from build123d import *

# Parameters (mm, degrees)
F0_W     = 4.7625
F0_H     = 3.175
F0_W_2   = 25.4
F0_H_2   = 4.7625
F1_DEPTH = 4.7625
F2_DEPTH = 25.4
F3_SIZE  = 6.35
F4_R     = 3.96875
F4_R_2   = 1.984375
F5_DEPTH = 0.79375
F6_DEPTH = 4.7625


with BuildPart() as f1:
    # F0 (on Top) → F1 (new body)
    with BuildSketch(Plane.XY):
        with Locations((27.78125, 17.0815)):
            Rectangle(F0_W, F0_H)
        with Locations((27.78125, -17.0815)):
            Rectangle(F0_W, F0_H)
        with Locations((-42.8625, -21.05025)):
            Rectangle(F0_W_2, F0_H_2)
        Polygon((25.4, -18.669), (-25.4, -18.669), (-30.1625, -18.669), (-30.1625, -23.4315), (30.1625, -23.4315), (30.1625, -18.669), align=None)
        Polygon((-25.4, 18.669), (25.4, 18.669), (30.1625, 18.669), (30.1625, 23.4315), (-30.1625, 23.4315), (-30.1625, -18.669), (-25.4, -18.669), align=None)
        Polygon((25.4, 15.494), (25.4, 18.669), (-25.4, 18.669), (-25.4, -18.669), (25.4, -18.669), (25.4, -15.494), (-22.225, -15.494), (-22.225, 15.494), align=None)
    extrude(amount=F1_DEPTH)

    # F0 (on Top) → F2 (join)
    with BuildSketch(Plane.XY):
        with Locations((-42.8625, -21.05025)):
            Rectangle(F0_W_2, F0_H_2)
        Polygon((25.4, -18.669), (-25.4, -18.669), (-30.1625, -18.669), (-30.1625, -23.4315), (30.1625, -23.4315), (30.1625, -18.669), align=None)
        Polygon((-25.4, 18.669), (25.4, 18.669), (30.1625, 18.669), (30.1625, 23.4315), (-30.1625, 23.4315), (-30.1625, -18.669), (-25.4, -18.669), align=None)
    extrude(amount=F2_DEPTH)

    # F3
    f3_edges = [f1.edges().sort_by_distance(p)[0] for p in [
        (-30.1625, -18.669, 12.7),
    ]]
    chamfer(f3_edges, length=F3_SIZE)

    # F4 (on face) → F5 (cut)
    with BuildSketch(Plane(origin=(0, -18.669, 0), x_dir=(-1, 0, 0), z_dir=(0, 1, 0))):
        with Locations((46.0375, 6.35)):
            Circle(F4_R)
        with Locations((46.0375, 6.35)):
            Circle(F4_R_2, mode=Mode.SUBTRACT)
        with Locations((46.0375, 19.05)):
            Circle(F4_R)
        with Locations((46.0375, 19.05)):
            Circle(F4_R_2, mode=Mode.SUBTRACT)
    extrude(amount=-F5_DEPTH, mode=Mode.SUBTRACT)

    # F6 (cut, through all): faces of the model
    f6_faces = [f1.faces().sort_by_distance(p)[0] for p in [
        (-46.0375, -18.669, 6.35),
        (-46.0375, -18.669, 19.05),
    ]]
    extrude(f6_faces, amount=-F6_DEPTH, mode=Mode.SUBTRACT)


solid = f1.part
The listing builds one solid part. Answer for the finished solid, in the listing's coordinates (mm). A direction names the side the tool comes from. Coordinates: 2 decimals unless noted, no trailing zeros. Write each loop counter-clockwise with the first axis right and the second up, starting at its lowest first coordinate (ties: lowest second). Pieces come first, ordered by that corner, then holes. Notation, with made-up numbers: (75, 40) - (80, 40) arc R11 ccw to (80, 59) - close; hole circle Ø4 at (39, -13). An arc over 180 degrees is marked (long way). Put each result on its own line as item: value.
1. The part is cut by section D-D on z = 3.5. Give the vertices of the cut face in (x, y) (1 decimal), plus the area to 3 significant figures.
Answer sheet:
outline: (-55.6, -23.4) - (30.2, -23.4) - (30.2, -15.5) - (-22.2, -15.5) - (-22.2, 15.5) - (30.2, 15.5) - (30.2, 23.4) - (-30.2, 23.4) - (-30.2, -12.3) - (-36.5, -18.7) - (-43.3, -18.7) - (-43.3, -19.5) - (-48.8, -19.5) - (-48.8, -18.7) - (-55.6, -18.7) - close
area: 1,340 mm^2
2. Find the intervals of material crossed by line 1 along Y through (x, z) = (-2, 8.5); line 2 along Z through (x, y) = (-21, -16); line 3 along Y through (x, z) = (-3, 4), in increasing order. Write a range as from..to.
Answer sheet:
line 1: y = -23.43..-18.67, 18.67..23.43
line 2: z = 0..4.76
line 3: y = -23.43..-15.49, 15.49..23.43
3. A tool of negligible diameter and unlimited length cuts with its end or side. For faces 5 (the face through (-22.4, -1.6, 0)), 6 (the face through (-25.4, 0, 15)), 7 (the face through (4, -15.494, 2)), 8 (the face through (-47.93, -21.42, 19.65)), 9 (the face through (-47, -19.463, 21)), from which of +Z, -Z, +X, -X, +Y, -Y can it reach the whole face along a straight path? Write none if from no direction.
Answer sheet:
face 5: -Z, +X, -X, +Y, -Y
face 6: +Z, +X
face 7: +Z, -Z, +X
face 8: +Y, -Y
face 9: +Y
4. The part is cut by section A-A on x = 16. Give the vertices of the cut face in (y, z).
Answer sheet:
outline: (-23.43, 0) - (-15.49, 0) - (-15.49, 4.76) - (-18.67, 4.76) - (-18.67, 25.4) - (-23.43, 25.4) - close; (15.49, 0) - (23.43, 0) - (23.43, 25.4) - (18.67, 25.4) - (18.67, 4.76) - (15.49, 4.76) - close
5. The part is cut by section C-C on y = -8.5. Give the vertices of the cut face in (x, z) (1 decimal).
Answer sheet:
outline: (-30.2, 0) - (-22.2, 0) - (-22.2, 4.8) - (-25.4, 4.8) - (-25.4, 25.4) - (-30.2, 25.4) - close
6. Determine the mould class of faces 1 (the face through (30.162, 20, 10)), 2 (the face through (-4, -17, 4.762)), 3 (the face through (-46, -18.669, 13)), 4 (the face through (-13, -23.432, 13)) for opening direction Y: pulls with the +Y half, pulls with the -Y half, needs draft (parallel to the pull), parting line crosses it, or undercut.
Answer sheet:
face 1: needs draft
face 2: undercut
face 3: pulls with the +Y half
face 4: pulls with the -Y half
7. The part is cut by section B-B on z = 19.05. Give the vertices of the cut face in (x, y).
Answer sheet:
outline: (-55.56, -23.43) - (-48.02, -23.43) - (-48.02, -19.46) - (-50.01, -19.46) - (-50.01, -18.67) - (-55.56, -18.67) - close; (-44.05, -23.43) - (30.16, -23.43) - (30.16, -18.67) - (-25.4, -18.67) - (-25.4, 18.67) - (30.16, 18.67) - (30.16, 23.43) - (-30.16, 23.43) - (-30.16, -12.32) - (-36.51, -18.67) - (-42.07, -18.67) - (-42.07, -19.46) - (-44.05, -19.46) - close
8. Flat-ended cylindrical pins translate along their axes: pin 1 Ø6 at (x, z) = (-41, 13.5) entering from +Y; pin 2 Ø5 at (x, z) = (-46.04, 19.05) entering from -Y; pin 3 Ø2 at (y, z) = (7.5, 5) entering from -X; pin 4 Ø2.5 at (x, z) = (-46, 7.5) entering from +Y. Find the tip coordinate at first contact, or state that the pin passes through.
Answer sheet:
pin 1: stops at y = -18.67
pin 2: stops at y = -23.43
pin 3: stops at x = -30.16
pin 4: stops at y = -19.46
